```python
from build123d import *

# Parameters (mm, degrees)
SKETCH_1_W          = 150
SKETCH_1_H          = 30
EXTRUDE_1_DEPTH     = 3
SKETCH_2_W          = 5
SKETCH_2_H          = 4.5
SKETCH_2_H_2        = 5
EXTRUDE_2_DEPTH     = 12
SKETCH_3_R          = 1.25
CUT_EXTRUDE_1_DEPTH = 12
CUT_EXTRUDE_2_DEPTH = 33
SKETCH_6_W          = 12
SKETCH_6_H          = 5
CUT_EXTRUDE_3_DEPTH = 14
CUT_EXTRUDE_4_DEPTH = 14
CUT_EXTRUDE_5_DEPTH = 14
SKETCH_9_W          = 52.537386277
SKETCH_9_H          = 169.005460475
CUT_EXTRUDE_6_DEPTH = 39


with BuildPart() as part:
    # 草图1 → 凸台-拉伸1 (new body)
    with BuildSketch(Plane(origin=(0, 0, 0), x_dir=(0, 0, -1), z_dir=(1, 0, 0))):
        with Locations((75, 15)):
            Rectangle(SKETCH_1_W, SKETCH_1_H)
    extrude_1 = extrude(amount=EXTRUDE_1_DEPTH)

    # 草图2 → 凸台-拉伸2 (add)
    with BuildSketch(Plane(origin=(3, 0, 0), x_dir=(0, 0, -1), z_dir=(1, 0, 0))):
        Polygon((6, 30), (11, 30), (11, 25.500001474), (6.003642258, 25.500001474), (6.003642258, 23.000001474), (11.003642258, 23.000001474), (11.003642258, 18.000001474), (6.003642258, 18.000001474), (6.003642258, 0), (0, 0), (0, 30), align=None)
        with Locations((36.5, 27.75)):
            Rectangle(SKETCH_2_W, SKETCH_2_H)
        with Locations((36.503642258, 20.500001474)):
            Rectangle(SKETCH_2_W, SKETCH_2_H_2)
    extrude_2 = extrude(amount=EXTRUDE_2_DEPTH)

    # 草图3 → 切除-拉伸1 (cut)
    with BuildSketch(Plane(origin=(0, 30, 0), x_dir=(1, 0, 0), z_dir=(0, 1, 0))):
        with Locations(Location((8.75, 36.25, 0), (0, 0, 270))):
            Circle(SKETCH_3_R)
        with Locations(Location((8.75, 8.75, 0), (0, 0, 270))):
            Circle(SKETCH_3_R)
    cut_extrude_1 = extrude(amount=-CUT_EXTRUDE_1_DEPTH, mode=Mode.SUBTRACT)

    # 草图5 → 切除-拉伸2 (cut)
    with BuildSketch(Plane(origin=(0, 30, 0), x_dir=(1, 0, 0), z_dir=(0, 1, 0))):
        with BuildLine():
            Line((0, 0), (9, 0))
            ThreePointArc((9, 0), (8.702388097, 0.045313059), (8.431747605, 0.17714569))
            Line((8.431747605, 0.17714569), (0, 6))
            Line((0, 6), (0, 0))
        make_face()
        with BuildLine():
            Line((15, 0), (15, 6))
            Line((15, 6), (9.733275958, 0.32006885))
            ThreePointArc((9.733275958, 0.32006885), (9.400043029, 0.083503642), (9, 0))
            Line((9, 0), (15, 0))
        make_face()
    cut_extrude_2 = extrude(amount=-CUT_EXTRUDE_2_DEPTH, mode=Mode.SUBTRACT)

    # 草图6 → 切除-拉伸3 (cut)
    with BuildSketch(Plane(origin=(0, 0, -6.003642258), x_dir=(-1, 0, 0), z_dir=(0, 0, -1))):
        with Locations((-9, 2.5)):
            Rectangle(SKETCH_6_W, SKETCH_6_H)
    cut_extrude_3 = extrude(amount=-CUT_EXTRUDE_3_DEPTH, mode=Mode.SUBTRACT)

    # 草图7 → 切除-拉伸4 (cut)
    with BuildSketch(Plane(origin=(3, 0, 0), x_dir=(0, 0, -1), z_dir=(1, 0, 0))):
        Polygon((41.659631445, 0), (3.928239346, 0), (3.928239346, 5), align=None)
    cut_extrude_4 = extrude(amount=-CUT_EXTRUDE_4_DEPTH, mode=Mode.SUBTRACT)

    # 草图8 → 切除-拉伸5 (cut)
    with BuildSketch(Plane(origin=(3, 0, 0), x_dir=(0, 0, -1), z_dir=(1, 0, 0))):
        with BuildLine():
            Line((100, 0), (150, 0))
            Line((150, 0), (150, 15))
            ThreePointArc((150, 15), (126.100766272, 3.830779092), (100, 0))
        make_face()
    cut_extrude_5 = extrude(amount=-CUT_EXTRUDE_5_DEPTH, mode=Mode.SUBTRACT)

    # 镜向2: 凸台-拉伸1, 凸台-拉伸2, 切除-拉伸1, 切除-拉伸2, 切除-拉伸3, 切除-拉伸4, 切除-拉伸5 across plane
    add(extrude_1.mirror(Plane(origin=(0, 0, 0), x_dir=(0, 0, 1), z_dir=(1, 0, 0))))
    add(extrude_2.mirror(Plane(origin=(0, 0, 0), x_dir=(0, 0, 1), z_dir=(1, 0, 0))))
    add(cut_extrude_1.mirror(Plane(origin=(0, 0, 0), x_dir=(0, 0, 1), z_dir=(1, 0, 0))), mode=Mode.SUBTRACT)
    add(cut_extrude_2.mirror(Plane(origin=(0, 0, 0), x_dir=(0, 0, 1), z_dir=(1, 0, 0))), mode=Mode.SUBTRACT)
    add(cut_extrude_3.mirror(Plane(origin=(0, 0, 0), x_dir=(0, 0, 1), z_dir=(1, 0, 0))), mode=Mode.SUBTRACT)
    add(cut_extrude_4.mirror(Plane(origin=(0, 0, 0), x_dir=(0, 0, 1), z_dir=(1, 0, 0))), mode=Mode.SUBTRACT)
    add(cut_extrude_5.mirror(Plane(origin=(0, 0, 0), x_dir=(0, 0, 1), z_dir=(1, 0, 0))), mode=Mode.SUBTRACT)

    # 草图9 → 切除-拉伸6 (cut)
    with BuildSketch(Plane(origin=(0, 30, 0), x_dir=(1, 0, 0), z_dir=(0, 1, 0))):
        with Locations((26.268693139, 84.502730238)):
            Rectangle(SKETCH_9_W, SKETCH_9_H)
    extrude(amount=-CUT_EXTRUDE_6_DEPTH, mode=Mode.SUBTRACT)


solid = part.part
```
The model under review builds one solid part; all positions refer to its coordinate system, in mm. A direction names the side the tool comes from. Coordinates: 2 decimals unless noted, no trailing zeros. Write each loop counter-clockwise with the first axis right and the second up, starting at its lowest first coordinate (ties: lowest second). Pieces come first, ordered by that corner, then holes. Notation, with made-up numbers: (19, 42.25) - (51, 42.25) arc R17 ccw to (51, 67.25) - close; hole circle Ø5 at (-24, 4). An arc over 180 degrees is marked (long way). Answer in a Markdown table with one row per item. Add a question column.
Q1. To check wall thickness, follow line 1 along Z through (x, y) = (-8.75, 26.55); line 2 along X through (y, z) = (27.5, -36.25); line 3 along X through (y, z) = (14.25, -30). State the ranges of each line that lie inside material, in increasing order. Write a range as from..to.
Q2. For faces 4 (the face through (-9, 20, -39.004)), 5 (the face through (-9, 5, -4)), 6 (the face through (-9, 12, -6.004)), 7 (the face through (-9, 23, -7)), list the 3-axis set-ups (+Z, -Z, +X, -X, +Y, -Y) from which the entire face can be reached by the end or side of a thin tool; tool diameter is ignored.
Q3. Consider section A-A on y = 21.25. Give the boundary of the cut face in (x, z).
Q4. Draft analysis for pull direction Y (two halves, no side actions). For faces 1 (the face through (-9, 18, -38)), 2 (the face through (-15, 26, -8)), 3 (the face through (-9, 23, -38)), state which applies: +Y half, -Y half, draft (parallel to the pull), parting line (faces both ways), or undercut.
Q5. Consider section C-C on x = -13.75. Give the boundary of the cut face in (y, z).
Q6. Consider section B-B on z = -36.25. Give the boundary of the cut face in (x, y), then the cut area to 3 significant figures.
Q7. Clearance check with flat-ended pins moving along their axes: pin 1 (3 mm diameter, centred on y = 17.5, z = -111, fed in from -X); pin 2 (5.5 mm diameter, centred on x = -8.5, z = -9, fed in from -Y); pin 3 (3 mm diameter, centred on x = -11.5, y = 9.5, fed in from -Z); pin 4 (1.5 mm diameter, centred on x = -9, z = -8.5, fed in from -Y). State where each tip first meets the part, or that it passes through.
Answers below:
| question | item | result |
|---|---|---|
| 1 | line 1 | -39..-37.5, -35..-34, -11..-10, -7.5..-0.03 |
| 1 | line 2 | -15..-10, -7.5..0 |
| 1 | line 3 | -3..0 |
| 2 | face 4 | -Z, -X, +Y, -Y |
| 2 | face 5 | +Z, -Z, -X, -Y |
| 2 | face 6 | -Z, -X, -Y |
| 2 | face 7 | -Z, -X |
| 3 | outline | (-15, -39) - (-3, -39) - (-3, -150) - (0, -150) - (0, -6) - (-8.43, -0.18) arc R1 ccw to (-9.73, -0.32) - (-15, -6) - (-15, -11) - (-3, -11) - (-3, -34) - (-15, -34) - close; hole circle Ø2.5 at (-8.75, -36.25); hole circle Ø2.5 at (-8.75, -8.75) |
| 4 | face 1 | -Y half |
| 4 | face 2 | draft |
| 4 | face 3 | undercut |
| 5 | outline | (5, -6) - (18, -6) - (18, -11) - (23, -11) - (23, -6) - (25.5, -6) - (25.5, -11) - (30, -11) - (30, -4.65) - (5, -4.65) - close; (18, -39) - (23, -39) - (23, -34) - (18, -34) - close; (25.5, -39) - (30, -39) - (30, -34) - (25.5, -34) - close |
| 6 | outline | (-15, 18) - (-10, 18) - (-10, 23) - (-15, 23) - close; (-15, 25.5) - (-10, 25.5) - (-10, 30) - (-15, 30) - close; (-7.5, 18) - (-3, 18) - (-3, 0.72) - (0, 0.72) - (0, 30) - (-7.5, 30) - (-7.5, 25.5) - (-3, 25.5) - (-3, 23) - (-7.5, 23) - close |
| 6 | area | 178 mm² |
| 7 | pin 1 | x = -3 |
| 7 | pin 2 | y = 18 |
| 7 | pin 3 | z = -6 |
| 7 | pin 4 | through |
